Part model, mm, in its own coordinate system. Coordinates: 2 decimals unless noted, no trailing zeros. Write each loop counter-clockwise with the first axis right and the second up, starting at its lowest first coordinate (ties: lowest second). Pieces come first, ordered by that corner, then holes. Notation, with made-up numbers: (-37.5, 0.5) - (-5.5, 0.5) arc R26 ccw to (-5.5, 20.5) - close; hole circle Ø5 at (69.5, 77). An arc over 180 degrees is marked (long way). Use one line per item in the form item = value. Start each with the question number.
Autodesk Inventor part; units mm, degrees
ref_plane "YZ Plane" through (0, 0, 0) normal (1, 0, 0) x (0, 1, 0)
ref_plane "XZ Plane" through (0, 0, 0) normal (0, 1, 0) x (-1, 0, 0)
ref_plane "XY Plane" through (0, 0, 0) normal (0, 0, 1) x (1, 0, 0)
sketch "Sketch1" plane through (0, 0, 0) normal (0, 0, 1) x (1, 0, 0)
  circle A0 centre (0, 0) radius 5.5499
  circle A1 centre (45.7905, 0) radius 2.0955
  circle A2 centre (26.8579, -16.9327) radius 2.0955
  arc A3 (0.9907, 9.4733) -> (-3.8129, -8.7285) centre (0, 0) ccw
  arc A4 (48.9628, -3.5521) -> (46.2858, 4.7367) centre (45.7905, 0) ccw
  arc A5 (24.9354, -21.2869) -> (30.0142, -20.4747) centre (26.8419, -16.9226) ccw
  line L0 (0.9907, 9.4733) -> (46.2858, 4.7367)
  line L1 (30.0142, -20.4747) -> (48.9628, -3.5521)
  line L2 (-3.8129, -8.7285) -> (24.9354, -21.2869)
  dimension "d0" = 11.0998
  dimension "d12" = 4.191
  dimension "d15" = 4.191
  dimension "d16" = 19.05
  dimension "d17" = 9.525
  dimension "d18" = 9.525
extrude "Extrusion1" add sketch "Sketch1" along normal blind 1.5875
sketch "Sketch2" plane through (0, 0, 1.5875) normal (0, 0, 1) x (1, 0, 0)
  circle A0 centre (3.175, -17.4625) radius 2.0828
  arc A1 (-1.5875, -17.4625) -> (5.2577, -21.7454) centre (3.175, -17.4625) ccw
  line L0 (-1.5875, -17.4625) -> (-1.5875, -11.7784)
  line L1 (-3.8129, -8.7285) -> (24.9354, -21.2869)
  arc A2 (-1.5875, -11.7784) -> (-3.4915, -8.8689) centre (-4.7625, -11.7784) ccw
  line L2 (5.2577, -21.7454) -> (13.7491, -17.6162)
  arc A3 (24.9354, -21.2869) -> (30.0142, -20.4747) centre (26.8419, -16.9226) ccw
  arc A4 (16.4085, -17.562) -> (13.7491, -17.6162) centre (15.1376, -20.4715) ccw
  point P0 (0, 0)
  point P1 (-1.5875, -9.7007)
  point P2 (15.0663, -16.9757)
  dimension "d19" = 4.1656
  dimension "d20" = 3.175
  dimension "d21" = 3.175
extrude "Extrusion2" add sketch "Sketch2" against normal blind 1.5875
properties part number "gear_gusset" material "Acetal Resin, White"
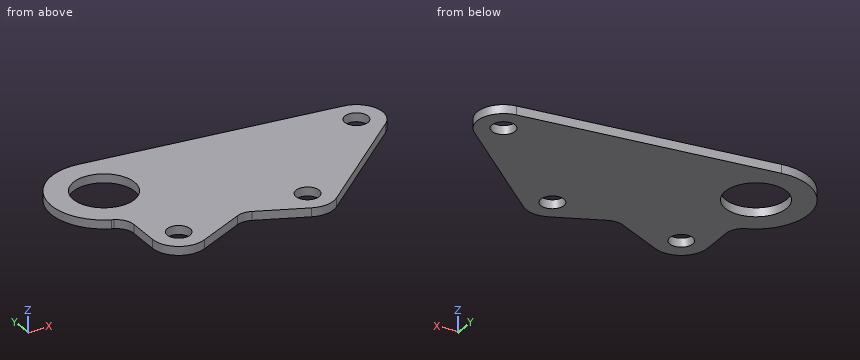
Q1. Slice it at D-D (x = 40). List the corners of the cut face in (y, z), plus the area to 3 significant figures.
Q2. Slice it at B-B (z = 0.25). Count the separate pieces of the cut face and the enclosed holes in it, plus the area to 3 significant figures.
Q3. Slice it at C-C (x = 0). List the corners of the cut face in (y, z), plus the area to 3 significant figures.
Q4. Pin check, flat tip, straight feed: P1, Ø4, axis at x = 9, y = -6.5, coming from the -Z side. Stop position of the tip, or through.
Q5. Drill centre lines: probe 1 along Y at (x, z) = (4, 0.55); probe 2 along X at (y, z) = (-3, 0.2); probe 3 along X at (y, z) = (-4.5, 1.3). Where is each one in solid material? Low to high.
Q6. Slice it at A-A (y = 0). List the corners of the cut face in (x, z) (1 decimal), plus the area to 3 significant figures.
Solution:
q1.outline = (-11.56, 0) - (5.39, 0) - (5.39, 1.59) - (-11.56, 1.59) - close
q1.area = 26.9 mm2
q2.separate_pieces = 1
q2.enclosed_holes = 4
q2.area = 1,200 mm2
q3.outline = (-21.01, 0) - (-5.55, 0) - (-5.55, 1.59) - (-21.01, 1.59) - close; (5.55, 0) - (9.52, 0) - (9.52, 1.59) - (5.55, 1.59) - close
q3.area = 30.9 mm2
q4.P1 = 0
q5.probe_1 = -22.15 to -19.37, -15.55 to -3.85, 3.85 to 9.16
q5.probe_2 = -9.04 to -4.67, 4.67 to 49.49
q5.probe_3 = -8.39 to -3.25, 3.25 to 47.9
q6.outline = (-9.5, 0) - (-5.5, 0) - (-5.5, 1.6) - (-9.5, 1.6) - close; (5.5, 0) - (43.7, 0) - (43.7, 1.6) - (5.5, 1.6) - close; (47.9, 0) - (50.6, 0) - (50.6, 1.6) - (47.9, 1.6) - close
q6.area = 71.1 mm2
